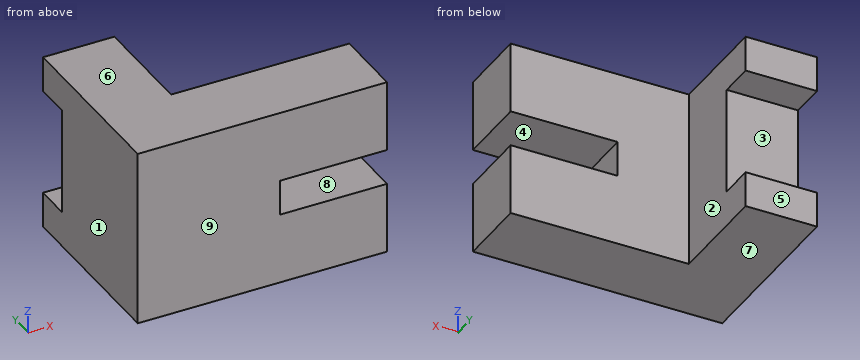
```python
from build123d import *

# Parameters (mm, degrees)
F1_DEPTH = 31.75
F2_W     = 12.7296627492
F2_H     = 19.05
F3_DEPTH = 6.35
F4_W     = 19.05
F4_H     = 6.35
F5_DEPTH = 14.4526


with BuildPart() as f1:
    # F0 (on Top) → F1 (new body)
    with BuildSketch(Plane.XY):
        Polygon((-31.7499138997, 0.0739416222), (-31.7499138997, 19.1239416222), (-44.4795766489, 19.1239416222), (-44.4795766489, -12.6999655599), (-0.0295766489, -12.6999655599), (0, 0), align=None)
    extrude(amount=F1_DEPTH)

    # F2 (on face) → F3 (cut)
    with BuildSketch(Plane(origin=(0, 19.1239416222, 0), x_dir=(-1, 0, 0), z_dir=(0, 1, 0))):
        with Locations((38.1147452743, 15.875)):
            Rectangle(F2_W, F2_H)
    extrude(amount=-F3_DEPTH, mode=Mode.SUBTRACT)

    # F4 (on face) → F5 (cut)
    with BuildSketch(Plane(origin=(0, 0, 0), x_dir=(-0.9999972882, 0.00232887, 0), z_dir=(0.00232887, 0.9999972882, 0))):
        with Locations((9.525, 15.875)):
            Rectangle(F4_W, F4_H)
    extrude(amount=-F5_DEPTH, mode=Mode.SUBTRACT)


solid = f1.part
```
Can you work these out from the model? Positions are in its coordinate system, mm. Face numbers are marked on the shaded views. A direction names the side the tool comes from. Coordinates: 2 decimals unless noted, no trailing zeros. Order: outer loops, then holes, each group sorted by start corner. A loop starts at its lowest first (then second) coordinate and runs counter-clockwise, first axis right, second up. Notation, with made-up numbers: (28, 78.25) -> (36, 78.25) arc R16 ccw to (36, 84.25) -> close; hole circle Ø8 at (23, -7.75). An arc over 180 degrees is marked (long way). Write each question's results on one line, items separated by ' | '.
Item 1: If we mould it in two halves opening along Z, with no side actions, what happens to the marked faces 6, 7, 8 and 9? For each: +Z half, -Z half, draft (parallel to the pull), parting line (faces both ways), or undercut.
Results are:
face 6: +Z half | face 7: -Z half | face 8: undercut | face 9: draft
Item 2: Which directions (+Z, -Z, +X, -X, +Y, -Y) give clear straight access to the entire face, cutting with the end or side of a thin tool? Please do the marked faces 1, 2, 3, 4 and 5.
Results are:
face 1: +Z, -Z, -X, +Y, -Y | face 2: +Z, -Z, +X, +Y | face 3: +X, -X, +Y | face 4: +X, +Y, -Y | face 5: +Z, -Z, +X, -X, +Y
Item 3: I'm going to push flat-ended pins straight in: pin 1 Ø4 at (x, z) = (-36.5, 16.5) entering from +Y; pin 2 Ø6.5 at (x, y) = (-12, -7) entering from -Z; pin 3 Ø5.5 at (y, z) = (5.5, 21.5) entering from +X. Where does each tip first touch, or does it pass through?
Results are:
pin 1: y = 12.77 | pin 2: z = 0 | pin 3: x = -31.75
Item 4: If I drill on line 1 along Z through (x, y) = (-41.5, 17.5); line 2 along Z through (x, y) = (-15.5, -6); line 3 along X through (y, z) = (7, 22), over which ranges is the centre line in solid material (lowest first)?
Results are:
line 1: 0 to 6.35, 25.4 to 31.75 | line 2: 0 to 12.7, 19.05 to 31.75 | line 3: -44.48 to -31.75
Item 5: I want a section at C-C, the plane z = 4.5. Write out the boundary of the cut face in (x, y).
Results are:
outline: (-44.48, -12.7) -> (-0.03, -12.7) -> (0, 0) -> (-31.75, 0.07) -> (-31.75, 19.12) -> (-44.48, 19.12) -> close
Item 6: I want a section at D-D, the plane y = -3.5. Write out the boundary of the cut face in (x, z), then the cut area to 3 significant figures.
Results are:
outline: (-44.48, 0) -> (-0.01, 0) -> (-0.01, 12.7) -> (-19.06, 12.7) -> (-19.06, 19.05) -> (-0.01, 19.05) -> (-0.01, 31.75) -> (-44.48, 31.75) -> close | area: 1,290 mm²
Item 7: I want a section at B-B, the plane x = -9.5. Write out the boundary of the cut face in (y, z).
Results are:
outline: (-12.7, 0) -> (0.02, 0) -> (0.02, 12.7) -> (-12.7, 12.7) -> close; (-12.7, 19.05) -> (0.02, 19.05) -> (0.02, 31.75) -> (-12.7, 31.75) -> close
Item 8: I want a section at A-A, the plane y = 13.5. Write out the boundary of the cut face in (x, z).
Results are:
outline: (-44.48, 0) -> (-31.75, 0) -> (-31.75, 6.35) -> (-44.48, 6.35) -> close; (-44.48, 25.4) -> (-31.75, 25.4) -> (-31.75, 31.75) -> (-44.48, 31.75) -> close
